from build123d import *

# Parameters (mm, degrees)
F0_W     = 30
F0_H     = 40
F1_DEPTH = 30
F2_W     = 20.5
F2_H     = 30
F3_DEPTH = 15
F4_W     = 34.05
F4_H     = 15
F5_DEPTH = 15
F6_R     = 4.25
F7_DEPTH = 25
F8_R     = 2
F9_DEPTH = 30.001
F10_R    = 3
F11_R    = 2


with BuildPart() as f1:
    # F0 (on Front) → F1 (new body)
    with BuildSketch(Plane.XZ):
        Rectangle(F0_W, F0_H)
    extrude(amount=F1_DEPTH)

    # F2 (on face) → F3 (cut)
    with BuildSketch(Plane.XZ.offset(30)):
        Rectangle(F2_W, F2_H)
    extrude(amount=-F3_DEPTH, mode=Mode.SUBTRACT)

    # F4 (on face) → F5 (cut)
    with BuildSketch(Plane.XZ.offset(30)):
        with Locations((2.025, 12.5)):
            Rectangle(F4_W, F4_H)
    extrude(amount=-F5_DEPTH, mode=Mode.SUBTRACT)

    # F6 (on face) → F7 (cut)
    with BuildSketch(Plane.XZ.offset(15)):
        Circle(F6_R)
    extrude(amount=-F7_DEPTH, mode=Mode.SUBTRACT)

    # F8 (on face) → F9 (cut, through all)
    with BuildSketch(Plane.YZ.offset(15)):
        with Locations((-20, -5)):
            Circle(F8_R)
    extrude(amount=-F9_DEPTH, mode=Mode.SUBTRACT)

    # F10
    f10_edges = [f1.edges().sort_by_distance(p)[0] for p in [
        (15, -7.5, 20),
        (12.625, -30, 5),
        (-12.625, -30, 5),
        (12.625, -15, 5),
        (-12.625, -15, 5),
        (-15, -7.5, 20),
        (-15, -15, -20),
        (15, -15, -20),
    ]]
    fillet(f10_edges, radius=F10_R)

    # F11
    f11_edges = [f1.edges().sort_by_distance(p)[0] for p in [
        (-10.25, -15, -5),
        (0, -15, -15),
        (10.25, -15, -5),
    ]]
    fillet(f11_edges, radius=F11_R)


solid = f1.part
Can you work these out from the model? Positions are in its coordinate system, mm. A direction names the side the tool comes from. Round coordinates to 2 decimals unless told otherwise and drop trailing zeros. Write each loop counter-clockwise with the first axis right and the second up, starting at its lowest first coordinate (ties: lowest second). Pieces come first, ordered by that corner, then holes. Notation, with made-up numbers: (-7, 22) - (21, 22) arc R22 ccw to (21, 32) - close; hole circle Ø2 at (64, 16). An arc over 180 degrees is marked (long way). Write each question's results on one line, items separated by ' | '. Start each with the question number.
1) Please list where these lines run through material, in increasing order: line 1 (Z direction, x = 0, y = -8.5); line 2 (Z direction, x = 11.45, y = -20); line 3 (Y direction, x = 11, z = 12.5).
2) Suppose I cut it at A-A (z = 0). List the corners of the cut face in (x, y) for me.
3) Which directions (+Z, -Z, +X, -X, +Y, -Y) give clear straight access to the entire face, cutting with the end or side of a thin tool? Please do faces 4 (the cylindrical face through (9.68, -15.6, -3.34)), 5 (the flat face through (-13, -23, 5)), 6 (the cylindrical face through (-14.14, -7.6, 19.1)).
4) We'd pull the mould along Y, two halves only. Please class faces 1 (the flat face through (-15, -15, -4)), 2 (the cylindrical face through (-9.68, -15.6, -3.66)), 3 (the cylindrical face through (-12.6, -21.6, -6.2)): released by +Y, released by -Y, zero draft, split by the parting line, or undercut.
5) For pin 1 Ø10.5 at (x, y) = (-2, -23) entering from +Z; pin 2 Ø5 at (x, z) = (0, 0) entering from +Y; pin 3 Ø3 at (x, z) = (-6, 7.5) entering from -Y; pin 4 Ø4 at (x, y) = (9.5, -23) entering from +Z, each with a flat end and sliding along its axis, tell me the tip position at first contact or that it passes through.
6) Suppose I cut it at B-B (y = -20). List the corners of the cut face in (x, z) for me.
7) Suppose I cut it at D-D (y = -11.5). List the corners of the cut face in (x, z) for me.
8) Suppose I cut it at C-C (x = 0). List the corners of the cut face in (y, z) for me, and give its area (3 significant figures).
Here are the results:
1) line 1: z = -20 to -4.25, 4.25 to 20 | line 2: z = -20 to -7, -3 to 5 | line 3: y = -15 to 0
2) outline: (-15, -30) - (-10.25, -30) - (-10.25, -17) arc R2 cw to (-8.25, -15) - (-4.25, -15) - (-4.25, 0) - (-15, 0) - close; (4.25, -15) - (8.25, -15) arc R2 cw to (10.25, -17) - (10.25, -30) - (15, -30) - (15, 0) - (4.25, 0) - close
3) face 4: +Z, -Y | face 5: +Z, +X, -X, -Y | face 6: +Z, -X, +Y, -Y
4) face 1: zero draft | face 2: released by -Y | face 3: undercut
5) pin 1: stops at z = -15 | pin 2: passes through | pin 3: stops at y = -15 | pin 4: stops at z = 5
6) outline: (-15, -17) arc R3 ccw to (-12, -20) - (12, -20) arc R3 ccw to (15, -17) - (15, -7) - (10.25, -7) - (10.25, -15) - (-10.25, -15) - (-10.25, -7) - (-15, -7) - close; (-15, -3) - (-10.25, -3) - (-10.25, 5) - (-15, 5) - close; (10.25, -3) - (15, -3) - (15, 5) - (10.25, 5) - close
7) outline: (-15, -17) arc R3 ccw to (-12, -20) - (12, -20) arc R3 ccw to (15, -17) - (15, 17) arc R3 ccw to (12, 20) - (-12, 20) arc R3 ccw to (-15, 17) - close; hole circle Ø8.5 at (0, 0)
8) outline: (-30, -20) - (0, -20) - (0, -4.25) - (-15, -4.25) - (-15, -13) arc R2 cw to (-17, -15) - (-30, -15) - close; (-15, 4.25) - (0, 4.25) - (0, 20) - (-15, 20) - close | area: 548 mm2
